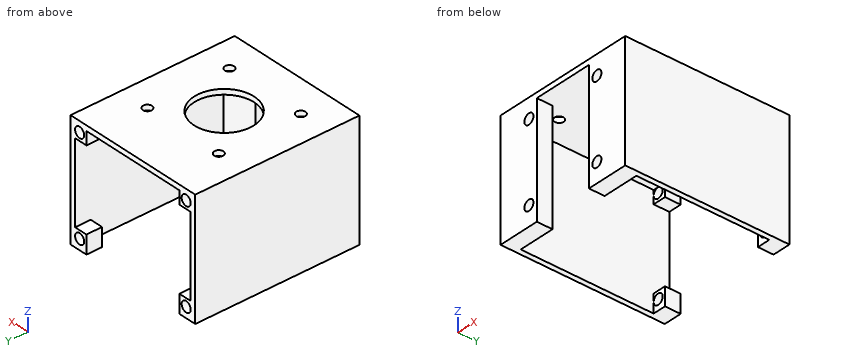
Autodesk Inventor part; units mm, degrees
ref_plane "YZ Plane" through (0, 0, 0) normal (1, 0, 0) x (0, 1, 0)
ref_plane "XZ Plane" through (0, 0, 0) normal (0, 1, 0) x (-1, 0, 0)
ref_plane "XY Plane" through (0, 0, 0) normal (0, 0, 1) x (1, 0, 0)
sketch "Skizze1" plane through (0, 0, 0) normal (0, 1, 0) x (-1, 0, 0)
  line L0 (-27.5, 22.5) -> (27.5, 22.5)
  line L1 (27.5, 22.5) -> (27.5, -22.5)
  line L2 (27.5, -22.5) -> (-27.5, -22.5)
  line L3 (-27.5, -22.5) -> (-27.5, 22.5)
  line L4 (0, -31.5) -> (0, 31.5)
  line L5 (38.5, 0) -> (-38.5, 0)
  point P0 (0, 0)
  dimension "d0" = 55
  dimension "d1" = 45
extrude "Extrusion1" add sketch "Skizze1" along normal blind 3
sketch "Skizze2" plane through (0, 3, 0) normal (0, 1, 0) x (1, 0, 0)
  line L0 (-27.5, 22.5) -> (-27.5, -22.5)
  line L1 (27.5, -22.5) -> (27.5, 22.5)
  line L2 (-27.5, -22.5) -> (27.5, -22.5)
  line L3 (27.5, -22.5) -> (27.5, -20.5)
  line L4 (27.5, -20.5) -> (-27.5, -20.5)
  line L5 (-27.5, -20.5) -> (-27.5, -22.5)
  point P0 (0, 0)
  dimension "d4" = 2
extrude "Extrusion2" add sketch "Skizze2" along normal blind 57
sketch "Skizze3" plane through (-27.5, 0, 22.5) normal (0, 0, 1) x (1, 0, 0)
  circle A0 centre (27.5, 25) radius 11.5
  line L0 (0, 0) -> (55, 0)
  line L1 (55, 0) -> (55, 60)
  circle A1 centre (43.25, 9.25) radius 1.75
  circle A2 centre (11.75, 9.25) radius 1.75
  circle A3 centre (11.75, 40.75) radius 1.75
  circle A4 centre (43.25, 40.75) radius 1.75
  line L2 (0, 60) -> (55, 60)
  line L3 (27.5, 60) -> (27.5, 0)
  line L4 (4.6208, 25) -> (55, 25)
  dimension "d7" = 23
  dimension "d10" = 3.5
  dimension "d11" = 3.5
  dimension "d12" = 3.5
  dimension "d13" = 3.5
  dimension "d17" = 31.5
  dimension "d48" = 0
extrude "Extrusion3" cut sketch "Skizze3" against normal up to surface (2 mm away) contours L4 L3 A0 | A0 L3 L4 | L3 L4 A0 | A0 L4 L3 | A1 | A2 | A3 | A4
sketch "Skizze10" plane through (0, 3, 0) normal (0, 1, 0) x (1, 0, 0)
  line L0 (27.5, -20.5) -> (27.5, 22.5)
  line L1 (27.5, 22.5) -> (-27.5, 22.5)
  line L2 (27.5, -20.5) -> (25.5, -20.5)
  line L3 (25.5, -20.5) -> (25.5, 22.5)
  line L4 (25.5, 22.5) -> (27.5, 22.5)
  line L5 (27.5, 22.5) -> (27.5, -20.5)
  line L6 (27.5, -20.5) -> (-27.5, -20.5)
  line L7 (-27.5, 22.5) -> (-25.5, 22.5)
  line L8 (-25.5, 22.5) -> (-25.5, -20.5)
  line L9 (-25.5, -20.5) -> (-27.5, -20.5)
  line L10 (-27.5, -20.5) -> (-27.5, 22.5)
  point P0 (0, 0)
  point P1 (-27.5, -20.5)
  dimension "d43" = 2
  dimension "d44" = 2
extrude "Extrusion6" add sketch "Skizze10" along normal blind 57 contours L2 L3 L1 L0 | L6 L10 L1 L8
sketch "Skizze11" plane through (0, 0, 0) normal (0, -1, 0) x (1, 0, 0)
  line L0 (27.5, 22.5) -> (27.5, -22.5)
  line L1 (-27.5, 22.5) -> (27.5, 22.5)
  line L2 (27.5, -22.5) -> (-27.5, -22.5)
  line L3 (-27.5, -22.5) -> (-27.5, 22.5)
  line L4 (-27.5, 22.5) -> (27.5, 22.5)
  line L5 (27.5, 22.5) -> (27.5, -22.5)
  point P0 (0, 0)
extrude "Extrusion7" add sketch "Skizze11" along normal blind 3
sketch "Skizze12" plane through (0, 3, 0) normal (0, 1, 0) x (1, 0, 0)
  circle A0 centre (15, -15) radius 2
  circle A1 centre (-15, -15) radius 2
  circle A2 centre (15, 15) radius 2
  circle A3 centre (-15, 15) radius 2
  line L0 (0, 31.5) -> (0, -31.5)
  line L1 (-38.5, 0) -> (38.5, 0)
  point P0 (0, 0)
  dimension "d52" = 4
  dimension "d53" = 4
  dimension "d54" = 4
  dimension "d55" = 4
  dimension "d56" = 30
  dimension "d57" = 30
extrude "Extrusion8" cut sketch "Skizze12" against normal up to surface (6 mm away)
sketch "Skizze13" plane through (0, 60, 0) normal (0, 1, 0) x (1, 0, 0)
  line L0 (25.5, -20.5) -> (20.5, -20.5)
  line L1 (20.5, -20.5) -> (20.5, -15.5)
  line L2 (20.5, -15.5) -> (25.5, -15.5)
  line L3 (25.5, -15.5) -> (25.5, -20.5)
  line L4 (-25.5, 22.5) -> (-25.5, -20.5)
  line L5 (-25.5, -20.5) -> (-20.5, -20.5)
  line L6 (-20.5, -20.5) -> (-20.5, -15.5)
  line L7 (-20.5, -15.5) -> (-25.5, -15.5)
  line L8 (-25.5, -15.5) -> (-25.5, -20.5)
  line L9 (25.5, 22.5) -> (20.5, 22.5)
  line L10 (20.5, 22.5) -> (20.5, 15.5)
  line L11 (20.5, 15.5) -> (25.5, 15.5)
  line L12 (25.5, 15.5) -> (25.5, 22.5)
  line L13 (25.5, 22.5) -> (-25.5, 22.5)
  line L14 (-25.5, 22.5) -> (-20.5, 22.5)
  line L15 (-20.5, 22.5) -> (-20.5, 15.5)
  line L16 (-20.5, 15.5) -> (-25.5, 15.5)
  line L17 (-25.5, 15.5) -> (-25.5, 22.5)
  point P0 (0, 0)
  point P1 (-25.5, -15.5)
  dimension "d60" = 5
  dimension "d61" = 5
  dimension "d62" = 5
  dimension "d63" = 5
  dimension "d64" = 5
  dimension "d65" = 7
  dimension "d66" = 5
  dimension "d67" = 7
sketch "Skizze15" plane through (0, -3, 0) normal (0, -1, 0) x (1, 0, 0)
  line L0 (-27.5, -22.5) -> (27.5, -22.5)
  line L1 (-25.5, 20.5) -> (25.5, 20.5)
  line L2 (11.5, -22.5) -> (-11.5, -22.5)
  line L3 (-11.5, -22.5) -> (-11.5, 20.5)
  line L4 (-11.5, 20.5) -> (11.5, 20.5)
  line L5 (11.5, 20.5) -> (11.5, -22.5)
  line L6 (0, 31.5) -> (0, -31.5)
  line L7 (-38.5, 0) -> (38.5, 0)
  circle A0 centre (15, -15) radius 2
  point P0 (0, 0)
  point P1 (11.5, 20.5)
  dimension "d94" = 1.5
extrude "Extrusion11" cut sketch "Skizze15" against normal up to surface (6 mm away) contours L3 L7 L6 L0 | L6 L7 L5 L0 | L3 L1 L6 L7 | L6 L1 L5 L7
extrude "Extrusion12" add sketch "Skizze13" against normal blind 6
sketch "Skizze16" plane through (0, 60, 0) normal (0, 1, 0) x (1, 0, 0)
  line L0 (38.5, 0) -> (-38.5, 0)
  line L1 (0, 31.5) -> (0, -31.5)
  circle A0 centre (23.5, -18.5) radius 2
  circle A1 centre (-23.5, -18.5) radius 2
  circle A2 centre (-23.5, 18.5) radius 2
  circle A3 centre (23.5, 18.5) radius 2
  line L2 (-27.5, -22.5) -> (27.5, -22.5)
  line L3 (27.5, -22.5) -> (27.5, 22.5)
  line L4 (27.5, 22.5) -> (20.5, 22.5)
  line L5 (-20.5, 22.5) -> (-27.5, 22.5)
  line L6 (-27.5, 22.5) -> (-27.5, -22.5)
  point P0 (0, 0)
  dimension "d100" = 4
  dimension "d101" = 4
  dimension "d102" = 4
  dimension "d103" = 4
  dimension "d104" = 4
  dimension "d105" = 4
  dimension "d106" = 4
  dimension "d107" = 4
  dimension "d108" = 4
  dimension "d109" = 4
  dimension "d110" = 4
  dimension "d111" = 4
extrude "Extrusion13" cut sketch "Skizze16" against normal up to surface (6 mm away) contours A0 | A1 | A2 | A3
properties part number "_3D-Druck"
Design review of the part built by this model. Coordinates are the model's own, in mm. Round coordinates to 2 decimals unless told otherwise and drop trailing zeros. Write each loop counter-clockwise with the first axis right and the second up, starting at its lowest first coordinate (ties: lowest second). Pieces come first, ordered by that corner, then holes.
Item 1: For pin 1 Ø3 at (x, z) = (-15, 15) entering from +Y; pin 2 Ø11 at (x, z) = (-18.5, 1) entering from +Y; pin 3 Ø12 at (x, y) = (-16.5, 29.5) entering from -Z, all flat-tipped, find the tip position at first contact; note any pin that passes through.
Item 2: Consider section D-D on y = 25. Give the boundary of the cut face in (x, z), and give its area (3 significant figures).
Item 3: Consider section A-A on z = 1. Give the boundary of the cut face in (x, y).
Item 4: Wall thickness on L1, parallel to Z at x = 23.5, y = 58.15; L2, parallel to Z at x = -15, y = 0.3; L3, parallel to X at y = -1, z = -15: over which ranges is each line inside the solid? List them lowest first.
Item 5: Consider section B-B on y = 49. Give the boundary of the cut face in (x, z), and give its area (3 significant figures).
Item 6: Consider section C-C on x = -10.5. Give the boundary of the cut face in (y, z).
Check values:
1. pin 1: passes through
1. pin 2: stops at y = 3
1. pin 3: stops at z = 20.5
2. outline: (-27.5, -22.5) - (-25.5, -22.5) - (-25.5, 20.5) - (-11.5, 20.5) - (-11.5, 22.5) - (-27.5, 22.5) - close; (11.5, 20.5) - (25.5, 20.5) - (25.5, -22.5) - (27.5, -22.5) - (27.5, 22.5) - (11.5, 22.5) - close
2. area: 236 mm2
3. outline: (-27.5, -3) - (-11.5, -3) - (-11.5, 3) - (-25.5, 3) - (-25.5, 60) - (-27.5, 60) - close; (11.5, -3) - (27.5, -3) - (27.5, 60) - (25.5, 60) - (25.5, 3) - (11.5, 3) - close
4. L1: z = -22.5 to -20.5, -16.5 to -15.5, 15.5 to 16.5, 20.5 to 22.5
4. L2: z = -22.5 to -17, -13 to 13, 17 to 22.5
4. L3: x = -27.5 to -17, -13 to -11.5, 11.5 to 13, 17 to 27.5
5. outline: (-27.5, -22.5) - (-25.5, -22.5) - (-25.5, 20.5) - (25.5, 20.5) - (25.5, -22.5) - (27.5, -22.5) - (27.5, 22.5) - (-27.5, 22.5) - close
5. area: 282 mm2
6. outline: (-3, 20.5) - (20.31, 20.5) - (20.31, 22.5) - (-3, 22.5) - close; (29.69, 20.5) - (60, 20.5) - (60, 22.5) - (29.69, 22.5) - close
